Could you check a few things on this model? Use its own coordinates, in mm. Face numbers are marked on the shaded views. A direction names the side the tool comes from. Coordinates: 2 decimals unless noted, no trailing zeros. Order: outer loops, then holes, each group sorted by start corner. A loop starts at its lowest first (then second) coordinate and runs counter-clockwise, first axis right, second up. Notation, with made-up numbers: (63.5, 36.5) -> (117.5, 36.5) arc R22 cw to (117.5, 73.5) -> close; hole circle Ø7 at (63, 88). An arc over 180 degrees is marked (long way). Use a Markdown table: item, result. Add a question column.
1) If we section it at A-A (x = 0): Write out the boundary of the cut face in (y, z), plus the area to 3 significant figures.
2) If I drill on L1, parallel to X at y = 5.25, z = 15; L2, parallel to X at y = 36, z = 0; L3, parallel to Y at x = -16.5, z = 7.5, over which ranges is the centre line in solid material (lowest first)? Write a range as [from, to].
3) If we section it at D-D (x = -40): Write out the boundary of the cut face in (y, z).
4) Thinking about a two-plate mould opening in X: for the marked faces 5, 6 and 7, which applies, +X half, -X half, draft (parallel to the pull), parting line (faces both ways), or undercut?
5) If we section it at C-C (y = 22): Write out the boundary of the cut face in (x, z), plus the area to 3 significant figures.
6) Will these pins go through, and if not, where does the flat tip stop? pin 1 Ø4 at (x, z) = (1, -11.5) entering from +Y; pin 2 Ø10.5 at (x, z) = (40, 15) entering from +Y; pin 3 Ø13 at (x, y) = (0, 22) entering from +Z.
7) Which directions (+Z, -Z, +X, -X, +Y, -Y) give clear straight access to the entire face, cutting with the end or side of a thin tool? Please do the marked faces 1, 2, 3 and 4.
8) If we section it at B-B (z = 2): Write out the boundary of the cut face in (x, y).
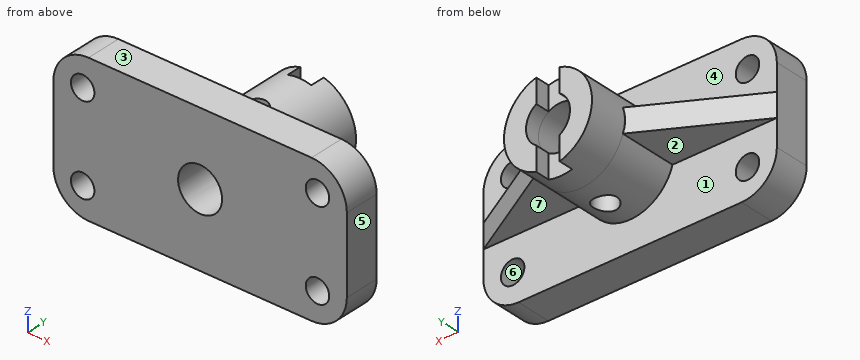
```python
from build123d import *

# Parameters (mm, degrees)
EXTRUDE_1_DEPTH          = 12
SKETCH_2_R               = 3.999999999999999
CUT_EXTRUDE_2_DEPTH      = 58.17516943569124
EXTRUDE_2_DEPTH          = 20
CUT_EXTRUDE_3_DEPTH      = 67.06814663663573
CUT_EXTRUDE_4_DEPTH      = 67.06814663663573
SKETCH_7_R               = 7.5
CUT_EXTRUDE_5_DEPTH      = 65.41273166075167
EXTRUDE_START            = -20
SKETCH_8_R               = 15
SKETCH_8_R_2             = 7.499999999999999
EXTRUDE_3_DEPTH          = 20
SKETCH_10_R              = 15
SKETCH_10_R_2            = 7.500000000000001
EXTRUDE_4_DEPTH          = 13
SKETCH_11_OUTSIDE_W      = 126.10400000000001
SKETCH_11_OUTSIDE_H      = 76.104
CUT_EXTRUDE_7_DEPTH      = 5
CUT_EXTRUDE_8_DEPTH      = 72.76350047203664
CUT_EXTRUDE_8_DEPTH_BACK = 72.76350047203664
SKETCH_12_R              = 4


with BuildPart() as part:
    # 草图1 → 凸台-拉伸1 (new body)
    with BuildSketch(Plane(origin=(0, 0, 0), x_dir=(1, 0, 0), z_dir=(0, 1, 0))):
        with BuildLine():
            Line((37.99999999999992, 25.00000000000001), (-37.999999999999915, 25))
            ThreePointArc((-37.999999999999915, 25), (-46.48528137423857, 21.485281374238575), (-50, 12.999999999999913))
            Line((-50, 12.999999999999913), (-49.99999999999999, -12.99999999999992))
            ThreePointArc((-49.99999999999999, -12.99999999999992), (-46.48528137423857, -21.48528137423858), (-37.99999999999991, -25.000000000000004))
            Line((-37.99999999999991, -25.000000000000004), (37.99999999999992, -24.999999999999993))
            ThreePointArc((37.99999999999992, -24.999999999999993), (46.48528137423858, -21.48528137423856), (50.00000000000001, -12.999999999999908))
            Line((50.00000000000001, -12.999999999999908), (50.00000000000001, 12.999999999999927))
            ThreePointArc((50.00000000000001, 12.999999999999927), (46.48528137423858, 21.485281374238582), (37.99999999999992, 25.00000000000001))
        make_face()
    extrude(amount=EXTRUDE_1_DEPTH)

    # 草图2 → 切除-拉伸2 (cut, through all)
    with BuildSketch(Plane(origin=(0, 12, 0), x_dir=(1, 0, 0), z_dir=(0, 1, 0))):
        with Locations(Location((-39.99999999999999, -15, 0), (0, 0, 270))):
            Circle(SKETCH_2_R)
        with Locations(Location((39.99999999999999, -15, 0), (0, 0, 90))):
            Circle(SKETCH_2_R)
        with Locations(Location((39.99999999999999, 15, 0), (0, 0, 270))):
            Circle(SKETCH_2_R)
        with Locations(Location((-39.99999999999999, 15, 0), (0, 0, 90))):
            Circle(SKETCH_2_R)
    extrude(amount=-CUT_EXTRUDE_2_DEPTH, mode=Mode.SUBTRACT)

    # 草图4 → 凸台-拉伸2 (add)
    with BuildSketch(Plane(origin=(0, 12, 0), x_dir=(1, 0, 0), z_dir=(0, 1, 0))):
        with BuildLine():
            Line((-50, -4), (-14.456832294800959, -4.000000000000001))
            ThreePointArc((-14.456832294800959, -4.000000000000001), (9.2e-16, -14.999999999999998), (14.456832294800959, -4))
            Line((14.456832294800959, -4), (50.00000000000001, -3.9999999999999982))
            Line((50.00000000000001, -3.9999999999999982), (50.00000000000001, 3.9999999999999982))
            Line((50.00000000000001, 3.9999999999999982), (14.456832294800959, 4))
            ThreePointArc((14.456832294800959, 4), (9.2e-16, 14.999999999999998), (-14.456832294800959, 4.000000000000001))
            Line((-14.456832294800959, 4.000000000000001), (-50, 4))
            Line((-50, 4), (-50, -4))
        make_face()
    extrude(amount=EXTRUDE_2_DEPTH)

    # 草图5 → 切除-拉伸3 (cut, through all)
    with BuildSketch(Plane.XY.offset(4.000000000000001)):
        Polygon((-14.456832294800959, 32), (-49.99999999999999, 12), (-50, 32), align=None)
    extrude(amount=-CUT_EXTRUDE_3_DEPTH, mode=Mode.SUBTRACT)

    # 草图6 → 切除-拉伸4 (cut, through all)
    with BuildSketch(Plane.XY.offset(4.000000000000001)):
        Polygon((14.456832294800959, 32), (50.00000000000001, 12), (50.00000000000001, 32), align=None)
    extrude(amount=-CUT_EXTRUDE_4_DEPTH, mode=Mode.SUBTRACT)

    # 草图7 → 切除-拉伸5 (cut, through all)
    with BuildSketch(Plane(origin=(0, 32, 0), x_dir=(1, 0, 0), z_dir=(0, 1, 0))):
        with Locations(Location((0, 0, 0), (0, 0, 270))):
            Circle(SKETCH_7_R)
    extrude(amount=-CUT_EXTRUDE_5_DEPTH, mode=Mode.SUBTRACT)

    # 草图8 → 凸台-拉伸3 (add)
    with BuildSketch(Plane(origin=(0, 32, 0), x_dir=(1, 0, 0), z_dir=(0, 1, 0)).offset(EXTRUDE_START)):
        Circle(SKETCH_8_R)
        with Locations(Location((0, 0, 0), (0, 0, 270))):
            Circle(SKETCH_8_R_2, mode=Mode.SUBTRACT)
    extrude(amount=EXTRUDE_3_DEPTH)

    # 草图10 → 凸台-拉伸4 (add)
    with BuildSketch(Plane(origin=(0, 32, 0), x_dir=(1, 0, 0), z_dir=(0, 1, 0))):
        with Locations(Location((0, 0, 0), (0, 0, 164.533990047))):
            Circle(SKETCH_10_R)
        with Locations(Location((0, 0, 0), (0, 0, 270))):
            Circle(SKETCH_10_R_2, mode=Mode.SUBTRACT)
    extrude(amount=EXTRUDE_4_DEPTH)

    # 草图11 outside → 切除-拉伸7 (cut)
    with BuildSketch(Plane(origin=(0, 45, 0), x_dir=(1, 0, 0), z_dir=(0, 1, 0))):
        Rectangle(SKETCH_11_OUTSIDE_W, SKETCH_11_OUTSIDE_H)
        with BuildLine():
            Line((4.000000000000002, -6.34428877022476), (4.000000000000003, -14.456832294800959))
            ThreePointArc((4.000000000000003, -14.456832294800959), (15, 0), (4.000000000000003, 14.456832294800959))
            Line((4.000000000000003, 14.456832294800959), (4.000000000000002, 6.34428877022476))
            ThreePointArc((4.000000000000002, 6.34428877022476), (7.500000000000001, 0), (4.000000000000002, -6.34428877022476))
        make_face(mode=Mode.SUBTRACT)
        with BuildLine():
            Line((-4.000000000000002, -6.34428877022476), (-4.000000000000003, -14.456832294800959))
            ThreePointArc((-4.000000000000003, -14.456832294800959), (-15, 1.84e-15), (-4.000000000000003, 14.456832294800959))
            Line((-4.000000000000003, 14.456832294800959), (-4.000000000000002, 6.34428877022476))
            ThreePointArc((-4.000000000000002, 6.34428877022476), (-7.500000000000001, 9.2e-16), (-4.000000000000002, -6.34428877022476))
        make_face(mode=Mode.SUBTRACT)
    extrude(amount=-CUT_EXTRUDE_7_DEPTH, mode=Mode.SUBTRACT)

    # 草图12 → 切除-拉伸8 (cut, two sides: drawn at the far end of the back side and taken through both)
    with BuildSketch(Plane.XY.offset(-CUT_EXTRUDE_8_DEPTH_BACK)):
        with Locations((0, 22)):
            Circle(SKETCH_12_R)
    extrude(amount=CUT_EXTRUDE_8_DEPTH + CUT_EXTRUDE_8_DEPTH_BACK, mode=Mode.SUBTRACT)


solid = part.part
```
Answer sheet:
| question | item | result |
|---|---|---|
| 1 | outline | (0, -25) -> (12, -25) -> (12, -15) -> (18, -15) -> (18, -7.5) -> (0, -7.5) -> close; (0, 7.5) -> (18, 7.5) -> (18, 15) -> (12, 15) -> (12, 25) -> (0, 25) -> close; (26, -15) -> (40, -15) -> (40, -7.5) -> (26, -7.5) -> close; (26, 7.5) -> (40, 7.5) -> (40, 15) -> (26, 15) -> close |
| 1 | area | 720 mm2 |
| 2 | L1 | [-49.83, -44], [-36, 36], [44, 49.83] |
| 2 | L2 | [-15, -7.5], [7.5, 15] |
| 2 | L3 | [0, 12] |
| 3 | outline | (0, -24.83) -> (12, -24.83) -> (12, -19) -> (0, -19) -> close; (0, -11) -> (12, -11) -> (12, -4) -> (17.63, -4) -> (17.63, 4) -> (12, 4) -> (12, 11) -> (0, 11) -> close; (0, 19) -> (12, 19) -> (12, 24.83) -> (0, 24.83) -> close |
| 4 | face 5 | +X half |
| 4 | face 6 | undercut |
| 4 | face 7 | draft |
| 5 | outline | (-32.23, -4) -> (-14.46, -4) arc R15 ccw to (-4, -14.46) -> (-4, -6.34) arc R7.5 cw to (-4, 6.34) -> (-4, 14.46) arc R15 ccw to (-14.46, 4) -> (-32.23, 4) -> close; (4, -14.46) arc R15 ccw to (14.46, -4) -> (32.23, -4) -> (32.23, 4) -> (14.46, 4) arc R15 ccw to (4, 14.46) -> (4, 6.34) arc R7.5 cw to (4, -6.34) -> close |
| 5 | area | 686 mm2 |
| 6 | pin 1 | y = 40 |
| 6 | pin 2 | y = 12 |
| 6 | pin 3 | z = 15 |
| 7 | face 1 | -Z, +Y |
| 7 | face 2 | -Z, -X, +Y |
| 7 | face 3 | +Z, +X, -X, +Y, -Y |
| 7 | face 4 | +Z, +Y |
| 8 | outline | (-50, 0) -> (-7.23, 0) -> (-7.23, 45) -> (-14.87, 45) -> (-14.87, 31.77) -> (-50, 12) -> close; (7.23, 0) -> (50, 0) -> (50, 12) -> (14.87, 31.77) -> (14.87, 45) -> (7.23, 45) -> close |
